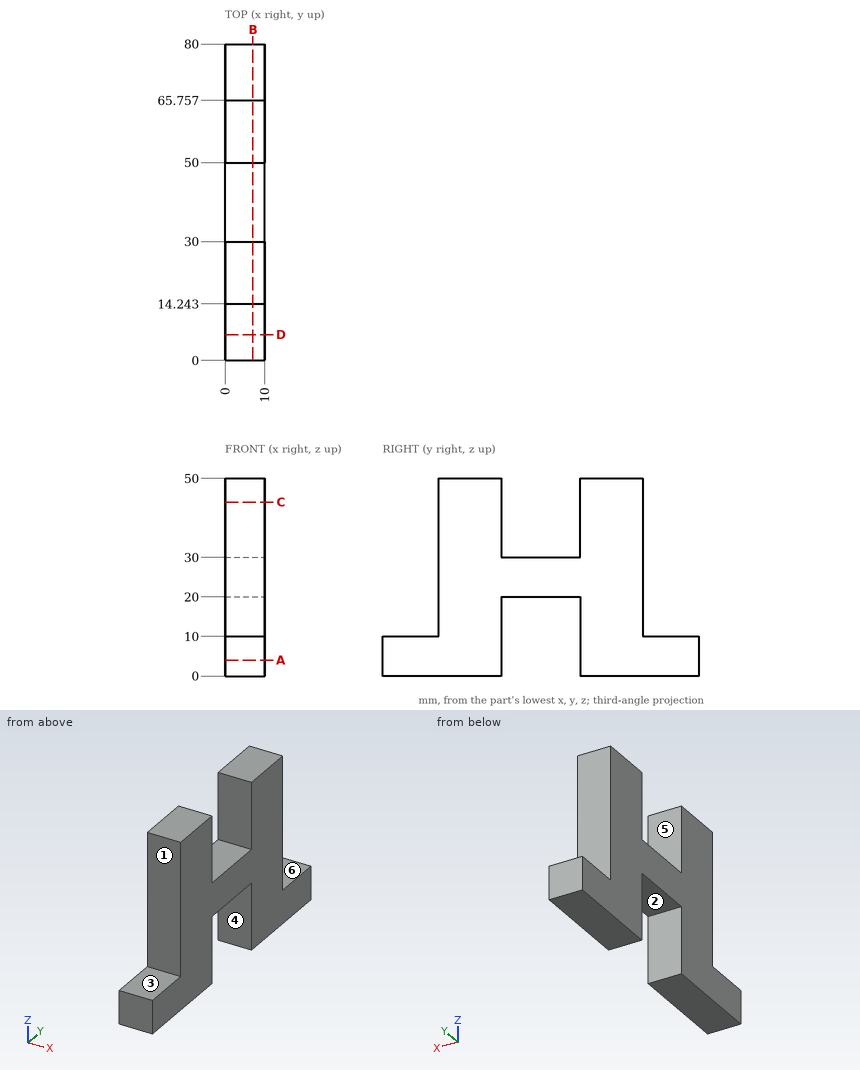
Job drawing, mm, ordinate dimensions from the low corner. One solid piece. A direction names the side the tool comes from. Coordinates: 2 decimals unless noted, no trailing zeros. Order: outer loops, then holes, each group sorted by start corner. A loop starts at its lowest first (then second) coordinate and runs counter-clockwise, first axis right, second up. Notation, with made-up numbers: (50, 25) -> (81, 25) arc R21 ccw to (81, 51) -> close; hole circle Ø1 at (10.25, 65). An arc over 180 degrees is marked (long way). Return JSON: item names as keys, results as strings. Group by question number.
Item 1: Tool access for the marked faces 4, 5 and 6: list every direction of +Z, -Z, +X, -X, +Y, -Y with a clear straight run to the whole face (end or side of a thin tool).
Item 2: Flat gauge pins, fed straight in: P1, Ø1.5, axis at x = 3, z = 15, coming from the +Y side; P2, Ø3, axis at x = 6, y = 40.5, coming from the -Z side; P3, Ø3, axis at x = 5.5, y = 43, coming from the +Z side. Where does each tip first touch, or does it go through?
Item 3: Pull direction Y, two halves, no side cores. Call the marked faces 1, 2 and 3: pulls with the +Y half, pulls with the -Y half, needs draft (parallel to the pull), parting line crosses it, or undercut.
Item 4: Saw through at A-A on z = 4. Write the cut outline in (x, y), then the cut area to 3 significant figures.
Item 5: Wall check: line 1 along Y through (x, z) = (3, 36.5); line 2 along Y through (x, z) = (4.25, 3); line 3 along Z through (x, y) = (3.5, 37). Give the ranges that are in metal, low to high. Write a range as [from, to].
Item 6: Saw through at B-B on x = 7. Write the cut outline in (y, z).
Item 7: Saw through at D-D on y = 6.5. Write the cut outline in (x, z).
Item 8: Saw through at C-C on z = 44. Write the cut outline in (x, y).
Values found:
{
 "1": {"face 4": "-Z, +X, -X", "face 5": "+Z, +X, -X", "face 6": "+Z, +X, -X, +Y"},
 "2": {"P1": "stops at y = 65.76", "P2": "stops at z = 20", "P3": "stops at z = 30"},
 "3": {"face 1": "pulls with the -Y half", "face 2": "undercut", "face 3": "needs draft"},
 "4": {"outline": "(0, 0) -> (10, 0) -> (10, 30) -> (0, 30) -> close; (0, 50) -> (10, 50) -> (10, 80) -> (0, 80) -> close", "area": "600 mm2"},
 "5": {"line 1": "y = [14.24, 30], [50, 65.76]", "line 2": "y = [0, 30], [50, 80]", "line 3": "z = [20, 30]"},
 "6": {"outline": "(0, 0) -> (30, 0) -> (30, 20) -> (50, 20) -> (50, 0) -> (80, 0) -> (80, 10) -> (65.76, 10) -> (65.76, 50) -> (50, 50) -> (50, 30) -> (30, 30) -> (30, 50) -> (14.24, 50) -> (14.24, 10) -> (0, 10) -> close"},
 "7": {"outline": "(0, 0) -> (10, 0) -> (10, 10) -> (0, 10) -> close"},
 "8": {"outline": "(0, 14.24) -> (10, 14.24) -> (10, 30) -> (0, 30) -> close; (0, 50) -> (10, 50) -> (10, 65.76) -> (0, 65.76) -> close"}
}
